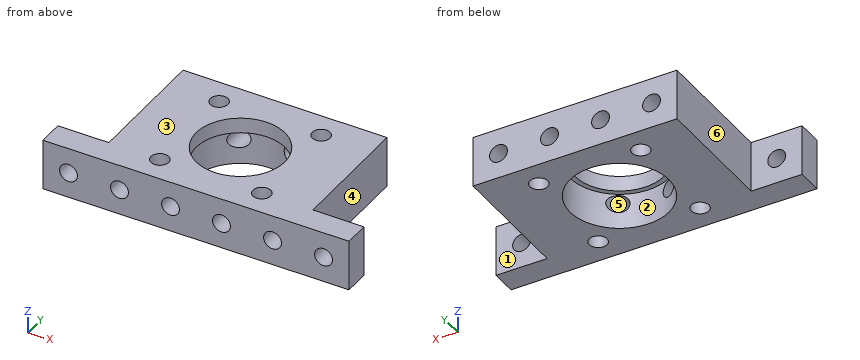
from build123d import *

# Parameters (mm, degrees)
ESQUISSE1_R             = 9.7
ESQUISSE1_R_2           = 1.75
BOSS_EXTRU_1_DEPTH      = 10
BOSS_EXTRU_2_START      = -3
ESQUISSE2_R             = 9.7
ESQUISSE2_R_2           = 8.7
BOSS_EXTRU_2_DEPTH      = 3
ESQUISSE3_R             = 1.75
ENL_V_MAT_EXTRU_1_DEPTH = 44.588989435


with BuildPart() as part:
    # Esquisse1 → Boss.-Extru.1 (new body)
    with BuildSketch(Plane.XY):
        Polygon((-20, -10), (-20, 15), (20, 15), (20, -10), (30, -10), (30, -15), (-30, -15), (-30, -10), align=None)
        Circle(ESQUISSE1_R, mode=Mode.SUBTRACT)
        with Locations((10, 10)):
            Circle(ESQUISSE1_R_2, mode=Mode.SUBTRACT)
        with Locations((-10, 10)):
            Circle(ESQUISSE1_R_2, mode=Mode.SUBTRACT)
        with Locations((-10, -10)):
            Circle(ESQUISSE1_R_2, mode=Mode.SUBTRACT)
        with Locations((10, -10)):
            Circle(ESQUISSE1_R_2, mode=Mode.SUBTRACT)
    extrude(amount=BOSS_EXTRU_1_DEPTH)

    # Esquisse2 → Boss.-Extru.2 (add)
    with BuildSketch(Plane.XY.offset(10).offset(BOSS_EXTRU_2_START)):
        Circle(ESQUISSE2_R)
        Circle(ESQUISSE2_R_2, mode=Mode.SUBTRACT)
    extrude(amount=BOSS_EXTRU_2_DEPTH)

    # Esquisse3 → Enlèv. mat.-Extru.1 (cut, through all)
    with BuildSketch(Plane.XZ.offset(15)):
        with Locations(Location((-25, 5, 0), (0, 0, 270))):
            Circle(ESQUISSE3_R)
        with Locations(Location((-15, 5, 0), (0, 0, 270))):
            Circle(ESQUISSE3_R)
        with Locations(Location((-5, 5, 0), (0, 0, 270))):
            Circle(ESQUISSE3_R)
        with Locations(Location((5, 5, 0), (0, 0, 270))):
            Circle(ESQUISSE3_R)
        with Locations(Location((15, 5, 0), (0, 0, 270))):
            Circle(ESQUISSE3_R)
        with Locations(Location((25, 5, 0), (0, 0, 270))):
            Circle(ESQUISSE3_R)
    extrude(amount=-ENL_V_MAT_EXTRU_1_DEPTH, mode=Mode.SUBTRACT)


solid = part.part
Build history of the part. All positions in model axes, mm. Face numbers are marked on the shaded views. A direction names the side the tool comes from. Give positions to 0.01 mm unless a question says otherwise; leave off trailing zeros. Loops run counter-clockwise (first coordinate to the right, second up) from the corner with the lowest first, then second, coordinate; pieces in that order, holes last. Notation, with made-up numbers: (59, 73) - (116, 73) arc R31 ccw to (116, 111) - close; hole circle Ø1 at (-15.5, -5). An arc over 180 degrees is marked (long way). Write item = value, one per line. Start each with the question number.
1) Band-saw the part on D-D on x = -26. Give the cut face in (y, z).
2) Pull direction Y, two halves, no side cores. Call the marked faces 1, 2 and 3: +Y half, -Y half, draft (parallel to the pull), parting line (faces both ways), or undercut.
3) Band-saw the part on C-C on x = 6. Give the cut face in (y, z), plus the area to 3 significant figures.
4) Drop a flat-ended pin along its axis: pin 1 Ø6 at (y, z) = (10, 3) entering from -X. Give the stop position or say it passes through.
5) Tool access for the marked faces 4, 5 and 6: list every direction of +Z, -Z, +X, -X, +Y, -Y with a clear straight run to the whole face (end or side of a thin tool).
6) Band-saw the part on B-B on z = 1.25. Give the cut face in (x, y).
7) Band-saw the part on A-A on y = 0. Give the cut face in (x, z).
8) Probe probe 1 along Y at (x, z) = (-10, 2.5); probe 2 along Y at (x, z) = (0, 1.25); probe 3 along Y at (x, z) = (0, 8.7). List the from-to ranges inside material, lowest first. Write a range as from..to.
Final values:
q1.outline = (-15, 0) - (-10, 0) - (-10, 3.56) - (-15, 3.56) - close; (-15, 6.44) - (-10, 6.44) - (-10, 10) - (-15, 10) - close
q2.face_1 = +Y half
q2.face_2 = undercut
q2.face_3 = draft
q3.outline = (-15, 0) - (-7.62, 0) - (-7.62, 3.56) - (-15, 3.56) - close; (-15, 6.44) - (-7.62, 6.44) - (-7.62, 7) - (-6.3, 7) - (-6.3, 10) - (-15, 10) - close; (6.3, 7) - (7.62, 7) - (7.62, 6.44) - (15, 6.44) - (15, 10) - (6.3, 10) - close; (7.62, 0) - (15, 0) - (15, 3.56) - (7.62, 3.56) - close
q3.area = 113 mm²
q4.pin_1 = -20
q5.face_4 = +Z, -Z, +X, +Y
q5.face_5 = +Y, -Y
q5.face_6 = +Z, -Z, -X, +Y
q6.outline = (-30, -15) - (30, -15) - (30, -10) - (20, -10) - (20, 15) - (-20, 15) - (-20, -10) - (-30, -10) - close; hole circle Ø3.5 at (-10, -10); hole circle Ø3.5 at (-10, 10); hole circle Ø19.4 at (0, 0); hole circle Ø3.5 at (10, -10); hole circle Ø3.5 at (10, 10)
q7.outline = (-20, 0) - (-9.7, 0) - (-9.7, 7) - (-8.7, 7) - (-8.7, 10) - (-20, 10) - close; (8.7, 7) - (9.7, 7) - (9.7, 0) - (20, 0) - (20, 10) - (8.7, 10) - close; hole circle Ø3.5 at (-15, 5); hole circle Ø3.5 at (15, 5)
q8.probe_1 = -15..-11.75, -8.25..8.25, 11.75..15
q8.probe_2 = -15..-9.7, 9.7..15
q8.probe_3 = -15..-8.7, 8.7..15
